Part model, mm, in its own coordinate system. Coordinates: 2 decimals unless noted, no trailing zeros. Order: outer loops, then holes, each group sorted by start corner. A loop starts at its lowest first (then second) coordinate and runs counter-clockwise, first axis right, second up. Notation, with made-up numbers: (55.5, -21.5) - (103.5, -21.5) arc R20 cw to (103.5, 4.5) - close; hole circle Ø5 at (53.25, -34). An arc over 180 degrees is marked (long way). Use a Markdown table: item, result. Add a question column.
1) Wall check: L1, parallel to X at y = 16, z = 12.7 (3 decimals); L2, parallel to Z at x = -25, y = 34; L3, parallel to X at y = 47, z = -12 (3 decimals). Give the ranges that are in metal, low to high. Write a range as [from, to].
2) Saw through at A-A on z = -12.7. Count the separate pieces of the cut face and the enclosed holes in it, then the cut area to 3 significant figures.
3) Drop a flat-ended pin along its axis: P1, Ø1, axis at x = -24.5, z = 0, coming from the -Y side. Give the stop position or say it passes through.
4) Saw through at B-B on y = 29.5. List the corners of the cut face in (x, z) (1 decimal), then the cut area to 3 significant figures.
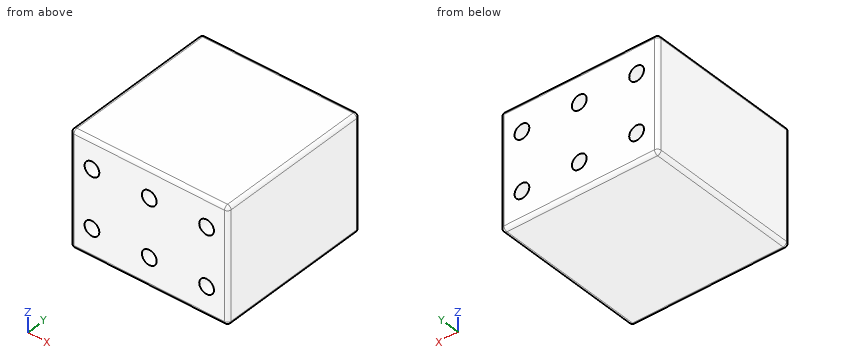
```python
from build123d import *

# Parameters (mm, degrees)
SKETCH1_W           = 69.85
SKETCH1_H           = 50.8
SKETCH1_R           = 3.2639
BOSS_EXTRUDE1_DEPTH = 69.85
FILLET1_R           = 1.5875


with BuildPart() as part:
    # Sketch1 → Boss-Extrude1 (new body)
    with BuildSketch(Plane(origin=(0, 0, 0), x_dir=(1, 0, 0), z_dir=(0, 1, 0))):
        Rectangle(SKETCH1_W, SKETCH1_H)
        with Locations(Location((-25.4, -12.7, 0), (0, 0, 270))):
            Circle(SKETCH1_R, mode=Mode.SUBTRACT)
        with Locations(Location((0, -12.7, 0), (0, 0, 270))):
            Circle(SKETCH1_R, mode=Mode.SUBTRACT)
        with Locations(Location((25.4, -12.7, 0), (0, 0, 270))):
            Circle(SKETCH1_R, mode=Mode.SUBTRACT)
        with Locations(Location((0, 12.7, 0), (0, 0, 270))):
            Circle(SKETCH1_R, mode=Mode.SUBTRACT)
        with Locations(Location((25.4, 12.7, 0), (0, 0, 270))):
            Circle(SKETCH1_R, mode=Mode.SUBTRACT)
        with Locations(Location((-25.4, 12.7, 0), (0, 0, 270))):
            Circle(SKETCH1_R, mode=Mode.SUBTRACT)
    extrude(amount=BOSS_EXTRUDE1_DEPTH)

    # Fillet1
    fillet1_edges = [part.edges().sort_by_distance(p)[0] for p in [
        (-34.925, 69.85, 0),
        (0, 69.85, 25.4),
        (34.925, 69.85, 0),
        (0, 0, 25.4),
        (-34.925, 0, 0),
        (0, 0, -25.4),
        (34.925, 0, 0),
        (34.925, 34.925, 25.4),
        (-34.925, 34.925, 25.4),
        (-34.925, 34.925, -25.4),
        (34.925, 34.925, -25.4),
        (0, 69.85, -25.4),
    ]]
    fillet(fillet1_edges, radius=FILLET1_R)


solid = part.part
```
Results are:
| question | item | result |
|---|---|---|
| 1 | L1 | [-34.925, -28.664], [-22.136, -3.264], [3.264, 22.136], [28.664, 34.925] |
| 1 | L2 | [-25.4, -15.94], [-9.46, 9.46], [15.94, 25.4] |
| 1 | L3 | [-34.925, -28.588], [-22.212, -3.188], [3.188, 22.212], [28.588, 34.925] |
| 2 | separate pieces | 4 |
| 2 | enclosed holes | 0 |
| 2 | area | 3,510 mm2 |
| 3 | P1 | y = 0 |
| 4 | outline | (-34.9, -23.8) arc R1.6 ccw to (-33.3, -25.4) - (33.3, -25.4) arc R1.6 ccw to (34.9, -23.8) - (34.9, 23.8) arc R1.6 ccw to (33.3, 25.4) - (-33.3, 25.4) arc R1.6 ccw to (-34.9, 23.8) - close; hole circle Ø6.5 at (-25.4, -12.7); hole circle Ø6.5 at (-25.4, 12.7); hole circle Ø6.5 at (0, -12.7); hole circle Ø6.5 at (0, 12.7); hole circle Ø6.5 at (25.4, -12.7); hole circle Ø6.5 at (25.4, 12.7) |
| 4 | area | 3,350 mm2 |
